The drawing under review shows one solid part. Ordinate dimensions are in mm from its lowest x, y, z. Round coordinates to 2 decimals unless told otherwise and drop trailing zeros. Order: outer loops, then holes, each group sorted by start corner. A loop starts at its lowest first (then second) coordinate and runs counter-clockwise, first axis right, second up.
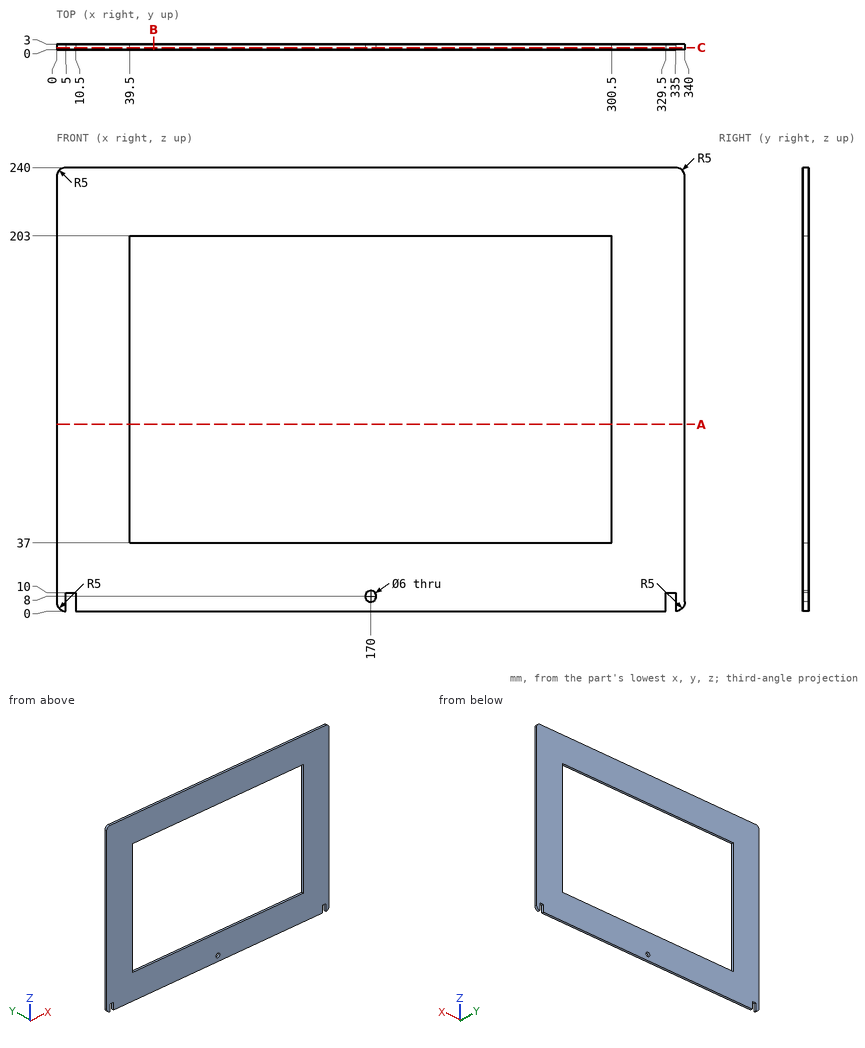
(1) We need section C-C (y = 1.1). Count the separate pieces of the cut face and the enclosed holes in it, and give its area (3 significant figures).
(2) Clearance check with flat-ended pins moving along their axes: P1, Ø0.9, axis at y = 1.5, z = 7.5, coming from the -X side; P2, Ø1.5, axis at x = 331, y = 1.5, coming from the -Z side. State where each tip first meets the part, or that it passes through.
(3) We need section A-A (z = 101). Give the boundary of the cut face in (x, y), and give its area (3 significant figures).
(4) We need section B-B (x = 52.5). Give the boundary of the cut face in (y, z), and give its area (3 significant figures).
(5) To check wall thickness, follow L1, parallel to Z at x = 170, y = 0.8; L2, parallel to Z at x = 177.5, y = 2.35; L3, parallel to X at y = 0.9, z = 119. State the ranges of each line that lie inside material, in increasing order.
Verdict:
1. separate pieces: 1
1. enclosed holes: 2
1. area: 38,100 mm2
2. P1: stops at x = 0
2. P2: stops at z = 10
3. outline: (0, 0) - (39.5, 0) - (39.5, 3) - (0, 3) - close; (300.5, 0) - (340, 0) - (340, 3) - (300.5, 3) - close
3. area: 237 mm2
4. outline: (0, 0) - (3, 0) - (3, 37) - (0, 37) - close; (0, 203) - (3, 203) - (3, 240) - (0, 240) - close
4. area: 222 mm2
5. L1: z = 0 to 5, 11 to 37, 203 to 240
5. L2: z = 0 to 37, 203 to 240
5. L3: x = 0 to 39.5, 300.5 to 340
